Autodesk Inventor part; units mm, degrees
ref_plane "YZ Plane" through (0, 0, 0) normal (1, 0, 0) x (0, 1, 0)
ref_plane "XZ Plane" through (0, 0, 0) normal (0, 1, 0) x (-1, 0, 0)
ref_plane "XY Plane" through (0, 0, 0) normal (0, 0, 1) x (1, 0, 0)
sketch "Sketch1" plane through (0, 0, 0) normal (0, 0, 1) x (1, 0, 0)
  line L0 (10.8649, 4.9355) -> (14.8649, 4.9355)
  line L1 (13.4649, 6.3355) -> (10.8649, 6.3355)
  line L2 (10.8649, 6.3355) -> (10.8649, 4.9355)
  line L3 (13.4649, 6.3355) -> (13.4649, 15.3355)
  line L4 (13.4649, 15.3355) -> (14.4649, 15.3355)
  line L5 (14.4649, 15.3355) -> (14.4649, 13.3355)
  line L6 (14.4649, 13.3355) -> (14.8649, 13.3355)
  line L7 (14.8649, 13.3355) -> (14.8649, 4.9355)
  line L8 (31.8649, 18.7517) -> (31.8649, 1.3446)
  dimension "d4" = 9
  dimension "d6" = 1
  dimension "d7" = 2
  dimension "d10" = 0.4
  dimension "d12" = 8.4
  dimension "d13" = 21
  dimension "d15" = 18.4
  dimension "d17" = 1.4
revolve "Revolution1" add sketch "Sketch1" angle 360 about axis through (31.8649, 18.7517, 0) along (0, -1, 0)
properties part number "mask_breath_top_lc"
The model under review builds one solid part; all positions refer to its coordinate system, in mm. A direction names the side the tool comes from. Give positions to 0.01 mm unless a question says otherwise; leave off trailing zeros. Write each loop counter-clockwise with the first axis right and the second up, starting at its lowest first coordinate (ties: lowest second). Pieces come first, ordered by that corner, then holes.
1. Add section D-D, the plane y = 14.75. Write out the cut boundary in (x, z).
2. Tool access review of faces 1 (the flat face through (24.2, 4.936, 15.5)), 2 (the cylindrical face through (50.247, 10.898, 0.809)): name each direction out of +Z, -Z, +X, -X, +Y, -Y from which nothing blocks a thin tool from reaching the whole face with its end or side.
3. For P1, Ø1.5, axis at y = 7, z = -4.5, coming from the -X side; P2, Ø6, axis at x = 28.5, y = 12, coming from the +Z side; P3, Ø1, axis at x = 36.5, y = 8.5, coming from the -Z side, all flat-tipped, find the tip position at first contact; note any pin that passes through.
4. Wall thickness on L1, parallel to X at y = 13.85, z = 0; L2, parallel to X at y = 9.75, z = 0; L3, parallel to Z at x = 32, y = 10.25: over which ranges is each line inside the solid? List them lowest first.
5. Add section C-C, the plane y = 7. Write out the cut boundary in (x, z).
6. Add section A-A, the plane z = 0. Write out the cut boundary in (x, y).
7. Draft analysis for pull direction Z (two halves, no side actions). For faces 3 (the cylindrical face through (11.835, 5.626, -6.308)), 4 (the flat face through (16.5, 13.336, 7.7)), 5 (the flat face through (32, 6.336, 19)), state which applies: +Z half, -Z half, draft (parallel to the pull), parting line (faces both ways), or undercut.
8. Add section B-B, the plane x = 23.5. Write out the cut boundary in (y, z), plus the area to 3 significant figures.
Worked answers:
1. outline: circle Ø36.8 at (31.86, 0); hole circle Ø34.8 at (31.86, 0)
2. face 1: +Z, -Z, +X, -X, -Y
2. face 2: +Y
3. P1: stops at x = 11.28
3. P2: stops at z = 18.4
3. P3: stops at z = -17.93
4. L1: x = 13.46 to 14.46, 49.26 to 50.26
4. L2: x = 13.46 to 14.86, 48.86 to 50.26
4. L3: z = -18.4 to -17, 17 to 18.4
5. outline: circle Ø36.8 at (31.86, 0); hole circle Ø34 at (31.86, 0)
6. outline: (10.86, 4.94) - (14.86, 4.94) - (14.86, 13.34) - (14.46, 13.34) - (14.46, 15.34) - (13.46, 15.34) - (13.46, 6.34) - (10.86, 6.34) - close; (48.86, 4.94) - (52.86, 4.94) - (52.86, 6.34) - (50.26, 6.34) - (50.26, 15.34) - (49.26, 15.34) - (49.26, 13.34) - (48.86, 13.34) - close
7. face 3: parting line
7. face 4: undercut
7. face 5: draft
8. outline: (4.94, -19.26) - (6.34, -19.26) - (6.34, -16.39) - (15.34, -16.39) - (15.34, -15.26) - (13.34, -15.26) - (13.34, -14.8) - (4.94, -14.8) - close; (4.94, 14.8) - (13.34, 14.8) - (13.34, 15.26) - (15.34, 15.26) - (15.34, 16.39) - (6.34, 16.39) - (6.34, 19.26) - (4.94, 19.26) - close
8. area: 39.3 mm2
